Could you check a few things on this drawing? It's one solid part, dimensions in mm from its lowest x, y, z. Give positions to 0.01 mm unless a question says otherwise; leave off trailing zeros. Loops run counter-clockwise (first coordinate to the right, second up) from the corner with the lowest first, then second, coordinate; pieces in that order, holes last. Notation, with made-up numbers: (24, 59) -> (52, 59) arc R25 cw to (52, 98) -> close; hole circle Ø5 at (-21, 58). An arc over 180 degrees is marked (long way). Use CSV: the item, a comma, the result in double quotes.
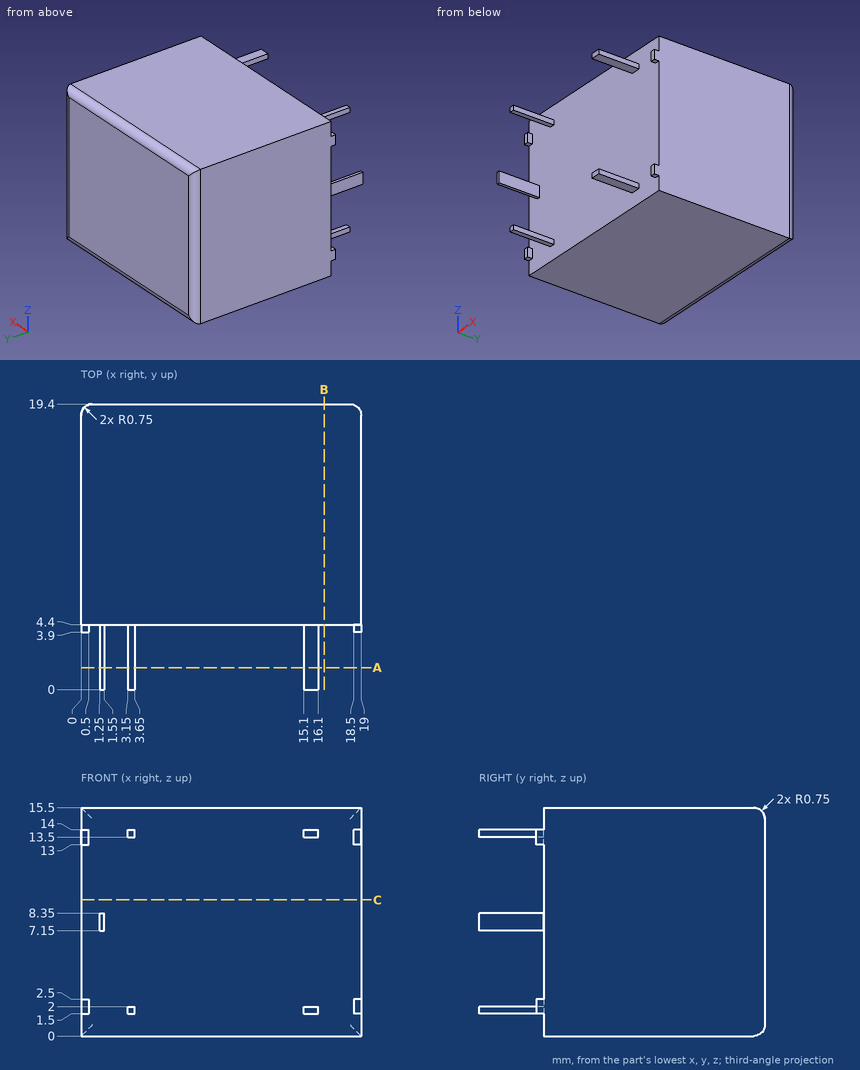
(1) Will these pins go through, and if not, where does the flat tip stop? pin 1 Ø0.6 at (x, y) = (3.5, 3) entering from -Z; pin 2 Ø3 at (x, z) = (4.5, 6.5) entering from -Y; pin 3 Ø0.6 at (y, z) = (1.5, 2) entering from -X.
Answer sheet:
pin 1,"stops at z = 1.5"
pin 2,"stops at y = 4.4"
pin 3,"stops at x = 3.15"
(2) If we section it at A-A, the plane y = 1.5: Write out the boundary of the cut face in (x, z).
Answer sheet:
outline,"(1.25, 7.15) -> (1.55, 7.15) -> (1.55, 8.35) -> (1.25, 8.35) -> close; (3.15, 1.5) -> (3.65, 1.5) -> (3.65, 2) -> (3.15, 2) -> close; (3.15, 13.5) -> (3.65, 13.5) -> (3.65, 14) -> (3.15, 14) -> close; (15.1, 1.5) -> (16.1, 1.5) -> (16.1, 2) -> (15.1, 2) -> close; (15.1, 13.5) -> (16.1, 13.5) -> (16.1, 14) -> (15.1, 14) -> close"
(3) If we section it at B-B, the plane x = 16.5: Write out the boundary of the cut face in (y, z), then the cut area to 3 significant figures.
Answer sheet:
outline,"(4.4, 0) -> (18.65, 0) arc R0.75 ccw to (19.4, 0.75) -> (19.4, 14.75) arc R0.75 ccw to (18.65, 15.5) -> (4.4, 15.5) -> close"
area,"232 mm2"
(4) If we section it at C-C, the plane z = 9.25: Write out the boundary of the cut face in (x, y).
Answer sheet:
outline,"(0, 4.4) -> (19, 4.4) -> (19, 18.65) arc R0.75 ccw to (18.25, 19.4) -> (0.75, 19.4) arc R0.75 ccw to (0, 18.65) -> close"
(5) If I drill on L1, parallel to Y at x = 1, z = 11.5, over which ranges is the centre line in solid material (lowest first)? Write a range as from..to.
Answer sheet:
L1,"y = 4.4..19.4"
